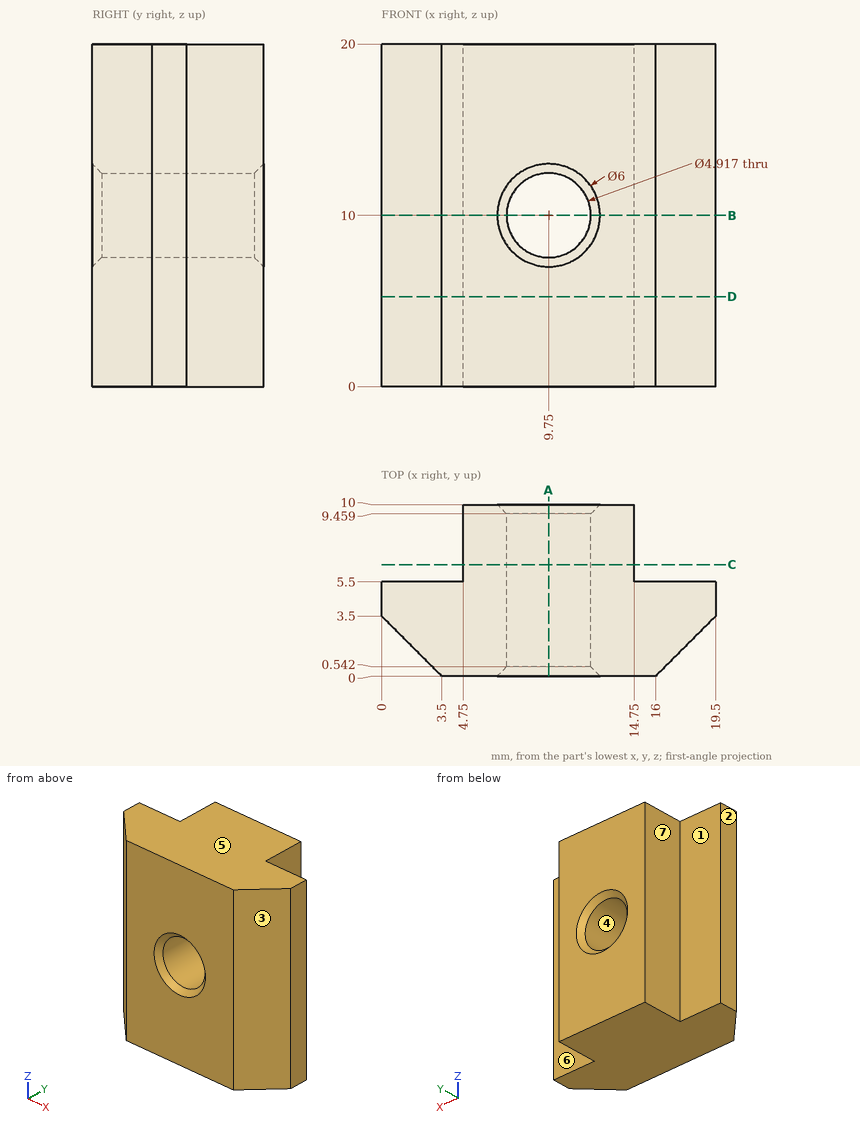
Here's the drawing with two shaded views (mm, measured from the low corner). I have some questions. A direction names the side the tool comes from. Round coordinates to 2 decimals unless told otherwise and drop trailing zeros. Loops run counter-clockwise (first coordinate to the right, second up) from the corner with the lowest first, then second, coordinate; pieces in that order, holes last.
Item 1: Suppose I cut it at B-B, the plane z = 10. Write out the boundary of the cut face in (x, y).
Item 2: If we mould it in two halves opening along X, with no side actions, what happens to the marked faces 1, 2, 3 and 4? For each: +X half, -X half, draft (parallel to the pull), parting line (faces both ways), or undercut.
Item 3: Please list where these lines run through material, in increasing order: L1, parallel to Z at x = 9.75, y = 7.75; L2, parallel to Y at x = 15.75, z = 14.5; L3, parallel to Z at x = 11.5, y = 3.75 (1 decimal).
Item 4: Suppose I cut it at A-A, the plane x = 9.75. Write out the boundary of the cut face in (y, z).
Item 5: Suppose I cut it at D-D, the plane z = 5.25. Write out the boundary of the cut face in (x, y), then the cut area to 3 significant figures.
Item 6: Suppose I cut it at C-C, the plane y = 6.5. Write out the boundary of the cut face in (x, z).
Item 7: Which directions (+Z, -Z, +X, -X, +Y, -Y) give clear straight access to the entire face, cutting with the end or side of a thin tool? Please do the marked faces 5, 6 and 7.
Item 8: Will these pins go through, and if not, where does the flat tip stop? pin 1 Ø1.3 at (y, z) = (7.5, 14) entering from +X; pin 2 Ø3 at (x, z) = (9.75, 10) entering from -Y; pin 3 Ø2.5 at (x, z) = (18, 6.5) entering from +Y; pin 4 Ø1 at (y, z) = (2.5, 16.5) entering from +X.
Reported:
1. outline: (0, 3.5) - (3.5, 0) - (6.75, 0) - (7.29, 0.54) - (7.29, 9.46) - (6.75, 10) - (4.75, 10) - (4.75, 5.5) - (0, 5.5) - close; (12.21, 0.54) - (12.75, 0) - (16, 0) - (19.5, 3.5) - (19.5, 5.5) - (14.75, 5.5) - (14.75, 10) - (12.75, 10) - (12.21, 9.46) - close
2. face 1: draft
2. face 2: -X half
2. face 3: +X half
2. face 4: undercut
3. L1: z = 0 to 7.54, 12.46 to 20
3. L2: y = 0 to 5.5
3. L3: z = 0 to 8.3, 11.7 to 20
4. outline: (0, 0) - (10, 0) - (10, 7) - (9.46, 7.54) - (0.54, 7.54) - (0, 7) - close; (0, 13) - (0.54, 12.46) - (9.46, 12.46) - (10, 13) - (10, 20) - (0, 20) - close
5. outline: (0, 3.5) - (3.5, 0) - (16, 0) - (19.5, 3.5) - (19.5, 5.5) - (14.75, 5.5) - (14.75, 10) - (4.75, 10) - (4.75, 5.5) - (0, 5.5) - close
5. area: 140 mm2
6. outline: (4.75, 0) - (14.75, 0) - (14.75, 20) - (4.75, 20) - close; hole circle Ø4.92 at (9.75, 10)
7. face 5: +Z, +X, -X, +Y, -Y
7. face 6: +Z, -Z, +X, +Y
7. face 7: +Z, -Z, -X, +Y
8. pin 1: stops at x = 14.75
8. pin 2: passes through
8. pin 3: stops at y = 5.5
8. pin 4: stops at x = 19
